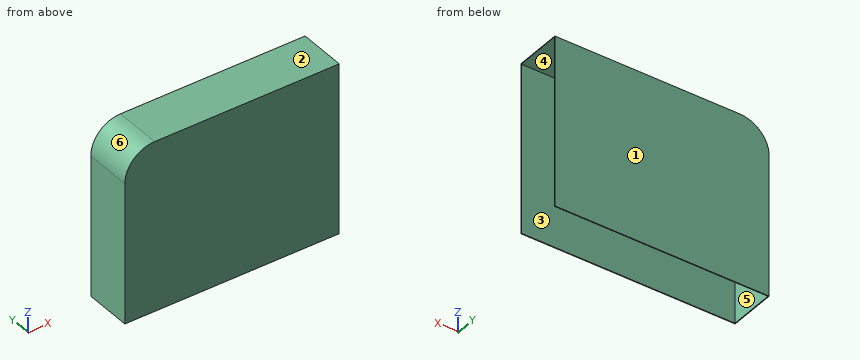
```python
from build123d import *

# Parameters (mm, degrees)
SALIENTE_EXTRUIR1_DEPTH = 32
VACIADO1_T              = -0.5
CROQUIS4_W              = 144.607899287
CROQUIS4_H              = 32
CORTAR_EXTRUIR2_DEPTH   = 3


with BuildPart() as part:
    # Croquis1 → Saliente-Extruir1 (new body)
    with BuildSketch(Plane(origin=(0, 0, 0), x_dir=(1, 0, 0), z_dir=(0, 1, 0))):
        with BuildLine():
            Line((20, 0), (144.607899287, 0))
            Line((144.607899287, 0), (144.607899287, 117.986152898))
            Line((144.607899287, 117.986152898), (0, 117.986152898))
            Line((0, 117.986152898), (0, 20))
            ThreePointArc((0, 20), (5.857864376, 5.857864376), (20, 0))
        make_face()
    extrude(amount=SALIENTE_EXTRUIR1_DEPTH)

    # Vaciado1
    vaciado1_openings = [part.faces().sort_by_distance(p)[0] for p in [
        (144.607899287, 16, -58.993076449),
    ]]
    offset(amount=VACIADO1_T, openings=vaciado1_openings, kind=Kind.INTERSECTION)

    # Croquis4 → Cortar-Extruir2 (cut)
    with BuildSketch(Plane(origin=(0, 0, -117.986152898), x_dir=(-1, 0, 0), z_dir=(0, 0, -1))):
        with Locations((-72.303949644, 16)):
            Rectangle(CROQUIS4_W, CROQUIS4_H)
    extrude(amount=-CORTAR_EXTRUIR2_DEPTH, mode=Mode.SUBTRACT)


solid = part.part
```
Geometry: final body of the model. Coordinates: model frame, mm. Face numbers are marked on the shaded views. A direction names the side the tool comes from. Coordinates: 2 decimals unless noted, no trailing zeros. Order: outer loops, then holes, each group sorted by start corner. A loop starts at its lowest first (then second) coordinate and runs counter-clockwise, first axis right, second up. Notation, with made-up numbers: (-14.5, -20.75) -> (41.5, -20.75) arc R35 cw to (41.5, 18.25) -> close; hole circle Ø11 at (29, -37.75). An arc over 180 degrees is marked (long way). Answer in a Markdown table with one row per item.
Item 1: Access query for the marked faces 5 and 6. Directions: +Z, -Z, +X, -X, +Y, -Y. A direction counts if a zero-diameter tool reaches every point of the face in a straight line with its end or side. Return the directions, or none.
Return value:
| item | result |
|---|---|
| face 5 | -Z, +X |
| face 6 | +Z, -X, +Y, -Y |
Item 2: Ray query, L1, parallel to Y at x = 26.5, z = -43; L2, parallel to Z at x = 50.5, y = 3; L3, parallel to X at y = 21, z = -46. Return the intervals inside material, ascending.
Return value:
| item | result |
|---|---|
| L1 | y = 0 to 0.5, 31.5 to 32 |
| L2 | z = -0.5 to 0 |
| L3 | x = 0 to 0.5 |
Item 3: Contact query for flat-ended pins moving along their axis: P1, Ø8, axis at x = 39.5, y = 15.5, coming from the -Z side; P2, Ø1.5, axis at y = 14, z = -39.5, coming from the +X side; P3, Ø10, axis at x = 20, y = 8.5, coming from the -Z side. Output: stop coordinate, or through.
Return value:
| item | result |
|---|---|
| P1 | stops at z = -0.5 |
| P2 | stops at x = 0.5 |
| P3 | stops at z = -1.15 |
Item 4: Draft query along Y for the marked faces 1, 2, 3 and 4. Return one class per face: released by +Y, released by -Y, zero draft, split by the parting line, or undercut.
Return value:
| item | result |
|---|---|
| face 1 | released by +Y |
| face 2 | zero draft |
| face 3 | undercut |
| face 4 | undercut |
Item 5: Section A-A on y = 20.5. Output: boundary loops of the cut face in (x, z), plus the area to 3 significant figures.
Return value:
| item | result |
|---|---|
| outline | (0, -114.99) -> (0.5, -114.99) -> (0.5, -20) arc R19.5 cw to (20, -0.5) -> (144.61, -0.5) -> (144.61, 0) -> (20, 0) arc R20 ccw to (0, -20) -> close |
| area | 125 mm² |
Item 6: Section B-B on z = -99. Output: boundary loops of the cut face in (x, y), plus the area to 3 significant figures.
Return value:
| item | result |
|---|---|
| outline | (0, 0) -> (144.61, 0) -> (144.61, 0.5) -> (0.5, 0.5) -> (0.5, 31.5) -> (144.61, 31.5) -> (144.61, 32) -> (0, 32) -> close |
| area | 160 mm² |
